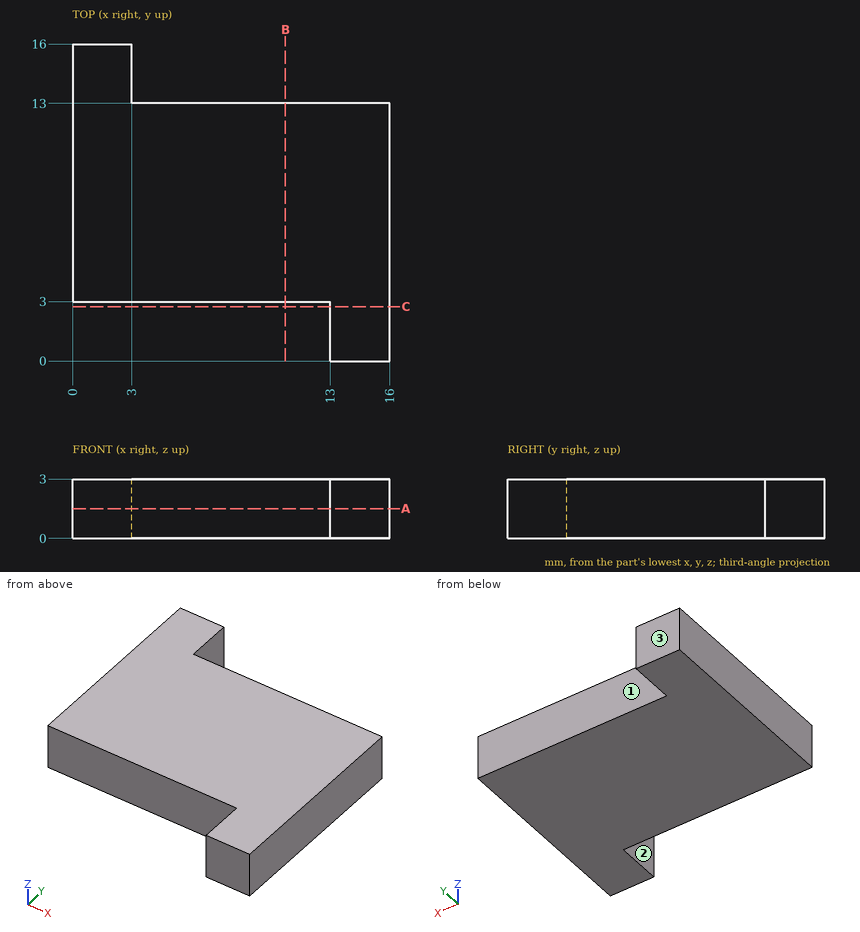
Answer from the drawing. Dimensions are ordinates in mm from the lowest x, y and z of the part. A direction names the side the tool comes from. Give positions to 0.01 mm unless a question says otherwise; leave off trailing zeros. Loops run counter-clockwise (first coordinate to the right, second up) from the corner with the lowest first, then second, coordinate; pieces in that order, holes last. Notation, with made-up numbers: (17.5, -7.5) - (31.5, -7.5) arc R22 cw to (31.5, 24.5) - close; hole circle Ø5 at (56, 23). An arc over 180 degrees is marked (long way). Write each question's results on one line, items separated by ' | '.
1. Find section B-B, the plane x = 10.75. Write down the section's boundary in (y, z), then the cut area to 3 significant figures.
Resolved:
outline: (3, 0) - (13, 0) - (13, 3) - (3, 3) - close | area: 30.0 mm^2
2. Find section A-A, the plane z = 1.5. Write down the section's boundary in (x, y).
Resolved:
outline: (0, 3) - (13, 3) - (13, 0) - (16, 0) - (16, 13) - (3, 13) - (3, 16) - (0, 16) - close
3. Which of the six approach directions +Z, -Z, +X, -X, +Y, -Y give full straight-line access (tool end or side, diameter ignored) to the marked faces 1, 2 and 3?
Resolved:
face 1: +Z, -Z, +X, +Y | face 2: +Z, -Z, -X, -Y | face 3: +Z, -Z, +X, -X, +Y
4. Consider probe 1 along Y at (x, z) = (9.5, 2.35); probe 2 along X at (y, z) = (15, 1.85); probe 3 along Y at (x, z) = (1.5, 0.3). Determine where each line is inside the solid, lowest interval first. Write a range as from..to.
Resolved:
probe 1: y = 3..13 | probe 2: x = 0..3 | probe 3: y = 3..16
5. Find section C-C, the plane y = 2.75. Write down the section's boundary in (x, z), then the cut area to 3 significant figures.
Resolved:
outline: (13, 0) - (16, 0) - (16, 3) - (13, 3) - close | area: 9.00 mm^2
